Source: CAD feature listing. Evaluate the final solid. Frame: model axes, mm. A direction names the side the tool comes from. Give positions to 0.01 mm unless a question says otherwise; leave off trailing zeros. Order: outer loops, then holes, each group sorted by start corner. A loop starts at its lowest first (then second) coordinate and runs counter-clockwise, first axis right, second up. Notation, with made-up numbers: M 78.5,28.5 L 122.5,28.5 A12 cw 122.5,45.5 Z; hole C 45.25,31 d5. An arc over 180 degrees is marked long. Answer in a Markdown table with one row per item. Add a question column.
(1) Section query D-D, the plane x = 36.5. Return loops of the section in (y, z), plus the area to 3 significant figures.
(2) Section query B-B, the plane x = 4. Return loops of the section in (y, z).
(3) Mould query, pull axis Z, two halves, no side actions, for faces 6 (the face through (47.465, -2.067, -9.152)), 7 (the face through (13.4, -17.43, -30.46)), 8 (the face through (-2.465, -2.615, -3.749)). Classes: pulls with the +Z half, pulls with the -Z half, needs draft (parallel to the pull), parting line crosses it, or undercut.
(4) Material intervals for line 1 along Z through (x, y) = (48.7, -5); line 2 along Z through (x, y) = (-1.2, -13); line 3 along Y through (x, z) = (-1, -4), sorted ascending.
(5) Section query C-C, the plane z = -21. Return loops of the section in (x, y), plus the area to 3 significant figures.
(6) Pin query (flat end, axial travel): P1, Ø1.5, axis at y = -6, z = -29.5, coming from the +X side; P2, Ø1.5, axis at x = 47.5, y = -8, coming from the -Z side. Return the tip coordinate at first contact, or that it passes through.
(7) Section query A-A, the plane z = -4.5. Return loops of the section in (x, y).
(8) Set-up query: faces 1 (the face through (47.465, -13.759, -7.917)), 2 (the face through (47, -9, -10)), 3 (the face through (33.5, -9.1, 3)), 4 (the face through (47.465, -16.007, -9.105)), 5 (the face through (22, -13, 0)). Return all of +Z, -Z, +X, -X, +Y, -Y with unobstructed straight access to the full face (end or side cutting, diameter ignored); none if empty.
from build123d import *

# Parameters (mm, degrees)
PAD004_DEPTH    = 18
POCKET001_DEPTH = 6.001
SKETCH009_R     = 2.5
POCKET002_DEPTH = 5.001
SKETCH020_W     = 5
SKETCH020_H     = 18
PAD011_DEPTH    = 10
SKETCH021_R     = 3.5
POCKET007_DEPTH = 5
POCKET008_DEPTH = 5
POCKET009_DEPTH = 5


with BuildPart() as part:
    # Sketch007 → Pad004 (new body)
    with BuildSketch(Plane.XZ):
        Polygon((0, 0), (45, 0), (50, 0), (50, 6), (-5, 6), (-5, -33), (14, -33), (14, -28), (0, -28), align=None)
    extrude(amount=PAD004_DEPTH)

    # Sketch008 → Pocket001 (cut, through all)
    with BuildSketch(Plane.XY):
        with BuildLine():
            ThreePointArc((16, -6.5), (13.5, -9), (16, -11.5))
            Line((16, -11.5), (31, -11.5))
            ThreePointArc((31, -11.5), (33.5, -9), (31, -6.5))
            Line((16, -6.5), (31, -6.5))
        make_face()
    extrude(amount=POCKET001_DEPTH, mode=Mode.SUBTRACT)

    # Sketch009 → Pocket002 (cut, through all)
    with BuildSketch(Plane.YZ):
        with Locations((-5, -4.5)):
            Circle(SKETCH009_R)
        with Locations((-13, -4.5)):
            Circle(SKETCH009_R)
    extrude(amount=-POCKET002_DEPTH, mode=Mode.SUBTRACT)

    # Sketch020 → Pad011 (join)
    with BuildSketch(Plane.XY):
        with Locations((47.5, -9)):
            Rectangle(SKETCH020_W, SKETCH020_H)
    extrude(amount=-PAD011_DEPTH)

    # Sketch021 → Pocket007 (cut)
    with BuildSketch(Plane.YZ.offset(45)):
        with Locations((-13, -4.5)):
            Circle(SKETCH021_R)
        with Locations((-5, -4.5)):
            Circle(SKETCH021_R)
    extrude(amount=POCKET007_DEPTH, mode=Mode.SUBTRACT)

    # Sketch022 → Pocket008 (cut)
    with BuildSketch(Plane.YZ.offset(45)):
        with BuildLine():
            ThreePointArc((-18, -6.791288), (-15.970515, -9.128827), (-13, -10))
            Line((-18, -10), (-13, -10))
            Line((-18, -6.791288), (-18, -10))
        make_face()
        with BuildLine():
            Line((0, -10), (0, -6.791288))
            ThreePointArc((-5, -10), (-2.029485, -9.128827), (0, -6.791288))
            Line((-5, -10), (0, -10))
        make_face()
    extrude(amount=POCKET008_DEPTH, mode=Mode.SUBTRACT)

    # Sketch023 → Pocket009 (cut)
    with BuildSketch(Plane.XY.offset(-28)):
        with BuildLine():
            ThreePointArc((12, -18), (13.414214, -17.414214), (14, -16))
            Line((14, -18), (14, -16))
            Line((12, -18), (14, -18))
        make_face()
        with BuildLine():
            ThreePointArc((14, -2), (13.414214, -0.585786), (12, 0))
            Line((14, 0), (12, 0))
            Line((14, -2), (14, 0))
        make_face()
    extrude(amount=-POCKET009_DEPTH, mode=Mode.SUBTRACT)


solid = part.part
Values follow:
| question | item | result |
|---|---|---|
| 1 | outline | M -18,0 L 0,0 L 0,6 L -18,6 Z |
| 1 | area | 108 mm² |
| 2 | outline | M -18,-33 L 0,-33 L 0,-28 L -18,-28 Z; M -18,0 L 0,0 L 0,6 L -18,6 Z |
| 3 | face 6 | pulls with the -Z half |
| 3 | face 7 | needs draft |
| 3 | face 8 | undercut |
| 4 | line 1 | z = -10 to -8, -1 to 6 |
| 4 | line 2 | z = -33 to -7, -2 to 6 |
| 4 | line 3 | y = -18 to -15.45, -10.55 to -7.45, -2.55 to 0 |
| 5 | outline | M -5,-18 L 0,-18 L 0,0 L -5,0 Z |
| 5 | area | 90.0 mm² |
| 6 | P1 | stops at x = 14 |
| 6 | P2 | stops at z = -10 |
| 7 | outline | M -5,-18 L 0,-18 L 0,-15.5 L -5,-15.5 Z; M -5,-10.5 L 0,-10.5 L 0,-7.5 L -5,-7.5 Z; M -5,-2.5 L 0,-2.5 L 0,0 L -5,0 Z; M 45,-18 L 50,-18 L 50,-16.5 L 45,-16.5 Z; M 45,-9.5 L 50,-9.5 L 50,-8.5 L 45,-8.5 Z; M 45,-1.5 L 50,-1.5 L 50,0 L 45,0 Z |
| 8 | face 1 | +X |
| 8 | face 2 | -Z, +X, +Y, -Y |
| 8 | face 3 | +Z, -Z |
| 8 | face 4 | -Z, +X, -Y |
| 8 | face 5 | +Y, -Y |
